from build123d import *

# Parameters (mm, degrees)
SKETCH1_W                = 79.618258269
SKETCH1_H                = 26
BOSS_EXTRUDE1_DEPTH      = 3
M3_CLEARANCE_HOLE1_D     = 3.4
M3_CLEARANCE_HOLE1_DEPTH = 5
M3_CLEARANCE_HOLE1_TIP   = 1.021463052
M3_CLEARANCE_HOLE2_D     = 3.4
M3_CLEARANCE_HOLE2_DEPTH = 5
M3_CLEARANCE_HOLE2_TIP   = 1.021463052
FILLET1_R                = 2


with BuildPart() as part:
    # Sketch1 → Boss-Extrude1 (new body)
    with BuildSketch(Plane.XY):
        with Locations((337.690870866, 0)):
            Rectangle(SKETCH1_W, SKETCH1_H)
    extrude(amount=BOSS_EXTRUDE1_DEPTH)

    # M3 Clearance Hole1
    with Locations(Plane.XY.offset(3)):
        with Locations((372, -7.5), (372, 7.5), (344, 7.5), (344, -7.5)):
            Hole(M3_CLEARANCE_HOLE1_D / 2, depth=M3_CLEARANCE_HOLE1_DEPTH)
            with Locations((0, 0, -(M3_CLEARANCE_HOLE1_DEPTH + M3_CLEARANCE_HOLE1_TIP / 2))):  # 118° drill point
                Cone(0, M3_CLEARANCE_HOLE1_D / 2, M3_CLEARANCE_HOLE1_TIP, mode=Mode.SUBTRACT)

    # M3 Clearance Hole2
    with Locations(Plane.XY.offset(3)):
        with Locations((309.046054969, 0), (327.046054969, 0)):
            Hole(M3_CLEARANCE_HOLE2_D / 2, depth=M3_CLEARANCE_HOLE2_DEPTH)
            with Locations((0, 0, -(M3_CLEARANCE_HOLE2_DEPTH + M3_CLEARANCE_HOLE2_TIP / 2))):  # 118° drill point
                Cone(0, M3_CLEARANCE_HOLE2_D / 2, M3_CLEARANCE_HOLE2_TIP, mode=Mode.SUBTRACT)

    # Fillet1
    fillet1_edges = [part.edges().sort_by_distance(p)[0] for p in [
        (297.881741731, 13, 1.5),
        (377.5, 13, 1.5),
        (377.5, -13, 1.5),
        (297.881741731, -13, 1.5),
    ]]
    fillet(fillet1_edges, radius=FILLET1_R)


solid = part.part
Model file for the job. Use its own axes, mm. Give positions to 0.01 mm unless a question says otherwise; leave off trailing zeros. Loops run counter-clockwise (first coordinate to the right, second up) from the corner with the lowest first, then second, coordinate; pieces in that order, holes last.
Item 1: Slice it at A-A (x = 344). Write the cut outline in (y, z), plus the area to 3 significant figures.
Check values:
outline: (-13, 0) - (-9.2, 0) - (-9.2, 3) - (-13, 3) - close; (-5.8, 0) - (5.8, 0) - (5.8, 3) - (-5.8, 3) - close; (9.2, 0) - (13, 0) - (13, 3) - (9.2, 3) - close
area: 57.6 mm2
Item 2: Drill centre lines: line 1 along Y through (x, z) = (372, 1.2); line 2 along X through (y, z) = (-1.25, 0.65); line 3 along X through (y, z) = (-8.5, 1.5). Where is each one in solid material? Low to high.
Check values:
line 1: y = -13 to -9.2, -5.8 to 5.8, 9.2 to 13
line 2: x = 297.88 to 307.89, 310.2 to 325.89, 328.2 to 377.5
line 3: x = 297.88 to 342.63, 345.37 to 370.63, 373.37 to 377.5
Item 3: Slice it at B-B (y = -7.5). Write the cut outline in (x, z), plus the area to 3 significant figures.
Check values:
outline: (297.88, 0) - (342.3, 0) - (342.3, 3) - (297.88, 3) - close; (345.7, 0) - (370.3, 0) - (370.3, 3) - (345.7, 3) - close; (373.7, 0) - (377.5, 0) - (377.5, 3) - (373.7, 3) - close
area: 218 mm2
Item 4: Slice it at C-C (z = 0.9). Write the cut outline in (x, y).
Check values:
outline: (297.88, -11) arc R2 ccw to (299.88, -13) - (375.5, -13) arc R2 ccw to (377.5, -11) - (377.5, 11) arc R2 ccw to (375.5, 13) - (299.88, 13) arc R2 ccw to (297.88, 11) - close; hole circle Ø3.4 at (309.05, 0); hole circle Ø3.4 at (327.05, 0); hole circle Ø3.4 at (344, -7.5); hole circle Ø3.4 at (344, 7.5); hole circle Ø3.4 at (372, -7.5); hole circle Ø3.4 at (372, 7.5)
Item 5: Mould opens along Y. For faces 1 (the face through (325.425, 0.511, 1.479)), 2 (the face through (298.452, -12.399, 1.521)), 3 (the face through (297.882, 0, 1)) say: +Y half, -Y half, draft (parallel to the pull), parting line (faces both ways), or undercut.
Check values:
face 1: undercut
face 2: -Y half
face 3: draft
